Source: CAD feature listing. Evaluate the final solid. Frame: model axes, mm. A direction names the side the tool comes from. Give positions to 0.01 mm unless a question says otherwise; leave off trailing zeros. Order: outer loops, then holes, each group sorted by start corner. A loop starts at its lowest first (then second) coordinate and runs counter-clockwise, first axis right, second up.
Autodesk Inventor part; units mm, degrees
ref_plane "Plano de trabajo4" through (-2.7452, -1.596, 0) normal (0, 0, -1) x (-1, 0, 0)
ref_plane "Plano de trabajo5" through (0, -3.175, 0) normal (0, 1, 0) x (-1, 0, 0)
ref_plane "Barreno" through (0, 0, 0) normal (0, -1, 0) x (1, 0, 0)
sketch "Boceto1" plane through (0, 0, 0) normal (0, 0, 1) x (1, 0, 0)
  line L0 (2.7452, 1.596) -> (2.7548, -1.5794)
  line L1 (2.7548, -1.5794) -> (0.0096, -3.1754)
  line L2 (0.0096, -3.1754) -> (-2.7452, -1.596)
  line L3 (-2.7452, -1.596) -> (-2.7548, 1.5794)
  line L4 (-2.7548, 1.5794) -> (-0.0096, 3.1754)
  line L5 (-0.0096, 3.1754) -> (2.7452, 1.596)
  point P0 (0, 0)
  point P1 (0, 0)
  dimension "d0" = 5.5
  dimension "d20" = 6.3508
extrude "Extrusión1" add sketch "Boceto1" along normal blind 15
ref_plane "Plano de trabajo4" through (-2.7452, -1.596, 0) normal (0, 0, -1) x (-1, 0, 0)
sketch "Boceto2" plane through (-2.7452, -1.596, 0) normal (0, 0, -1) x (-1, 0, 0)
  line L0 (-2.7548, -1.5794) -> (1.0358, -1.5794)
  line L1 (1.0358, -1.5794) -> (-2.7548, -1.5794)
  line L2 (-5.6299, -1.5794) -> (-2.7548, -1.5794)
  point P0 (-2.7452, 1.596)
  dimension "d5" = 3.1754
ref_plane "Plano de trabajo5" through (0, -3.175, 0) normal (0, 1, 0) x (-1, 0, 0)
sketch "Boceto3" plane through (0, -3.175, 0) normal (0, 1, 0) x (-1, 0, 0)
  line L0 (-0.0096, 15) -> (-2.7548, 15)
  line L1 (2.6199, 14) -> (-2.7548, 14) construction
  line L2 (-0.0096, 0) -> (-0.0096, 15)
  line L3 (-0.0096, 14) -> (-0.0096, 18.5)
  circle A0 centre (-0.0096, 18.5) radius 4.25
  circle A1 centre (-0.0096, 18.5) radius 2.75
  point P0 (0, 0)
  dimension "d7" = 1
  dimension "d8" = 4.5
  dimension "d9" = 8.5
  dimension "d14" = 5.5
sketch "Boceto4" plane through (-2.7452, -1.596, 0) normal (0, 0, -1) x (-1, 0, 0)
  point P0 (-2.7452, 1.596)
  point P1 (-2.7356, 4.7714)
  point P2 (-2.7548, -1.579)
  dimension "d10" = 6.3504
extrude "Extrusión2" add sketch "Boceto3" along normal blind 6.35 contours L2 A0 L0 | L0 A0 L2 | A1
ref_plane "Barreno" through (0, 0, 0) normal (0, -1, 0) x (1, 0, 0)
sketch "Boceto6" plane through (0, 0, 0) normal (0, -1, 0) x (1, 0, 0)
  arc A0 (0.0103, 14.25) -> (0.0089, 14.25) centre (0.0096, 18.5) ccw
  circle A1 centre (0.0096, 18.5) radius 2.75
  point P0 (0, 0)
  dimension "d13" = 4.25
extrude "Extrusión3" cut sketch "Boceto6" along normal mid plane 10 contours A1
ref_plane "Plano de trabajo8" through (5, 0, 0) normal (1, 0, 0) x (0, 1, 0)
sketch "Boceto8" plane through (5, 0, 0) normal (1, 0, 0) x (0, 1, 0)
  line L0 (-3.175, 15.75) -> (-3.175, 21.25)
  line L1 (-3.1754, 14.25) -> (-1.5794, 15)
  line L2 (-1.5794, 15) -> (-1.5794, 22.75)
  line L3 (-1.5794, 22.75) -> (-3.175, 22.75)
  line L4 (3.175, 14.25) -> (1.596, 15)
  line L5 (1.596, 15) -> (1.596, 22.75)
  line L6 (1.596, 22.75) -> (3.175, 22.75)
  ellipse E0 centre (3.1866, 18.5) end of major axis (3.1866, 14.25) minor radius 2.4709 (1.7849, 15) -> (3.175, 14.25) ccw
  line L7 (-3.175, 22.75) -> (-6.1952, 22.75)
  line L8 (-6.1952, 22.75) -> (-6.1952, 14.0055)
  line L9 (-6.1952, 14.0055) -> (-3.1754, 14.25)
  line L10 (3.175, 14.25) -> (7.2865, 13.4418)
  line L11 (7.2865, 13.4418) -> (6.5328, 22.75)
  line L12 (6.5328, 22.75) -> (3.175, 22.75)
  point P0 (0, 0)
  point P1 (-1.5794, 15)
extrude "Extrusión4" cut sketch "Boceto8" against normal blind 10 contours L9 L8 L7 L3 L2 L1 | L4 L5 L6 L12 L11 L10
fillet "Empalme1" radius 2 1 edges at (-2.75, 0, 15)
fillet "Empalme2" radius 2 1 edges at (2.75, 0.0083, 15)
ref_plane "Plano de trabajo9" through (0, 0, 0) normal (0, 0, -1) x (-1, 0, 0)
sketch "Boceto9" plane through (0, 0, 0) normal (0, 0, -1) x (-1, 0, 0)
  circle A0 centre (0, 0) radius 2.75
  line L0 (2.7548, 1.5794) -> (2.7452, -1.596)
extrude "Extrusión5" add sketch "Boceto9" along normal blind 0.01
properties part number "Cabezal" material "Plástico ABS"
1) Section query A-A, the plane z = 18.5. Return the cut outline in (x, y).
Report:
outline: (-4.24, -1.58) - (-2.74, -1.58) - (-2.74, 1.6) - (-4.24, 1.6) - close; (2.76, -1.58) - (4.26, -1.58) - (4.26, 1.6) - (2.76, 1.6) - close
2) Section query D-D, the plane z = 4.5. Return the cut outline in (x, y), and give its area (3 significant figures).
Report:
outline: (-2.75, -1.6) - (0.01, -3.18) - (2.75, -1.58) - (2.75, 1.6) - (-0.01, 3.18) - (-2.75, 1.58) - close
area: 26.2 mm2
3) Pin query (flat end, axial travel): pin 1 (3.5 mm diameter, centred on x = 0.01, z = 18.5, fed in from +Y). Return the tip coordinate at first contact, or that it passes through.
Report:
pin 1: passes through
4) Reachability of faces 1 (the flat face through (-1.349, -2.397, 7.353)), 2 (the flat face through (1.349, 2.397, 7.358)), 3 (the flat face through (-1.401, 2.366, 7.358)), 4 (the flat face through (0.1, -1.579, 21.4)) from +Z, -Z, +X, -X, +Y, -Y: full face, straight path, thin tool, end or side. Return the list, or none.
Report:
face 1: -Z, -X, -Y
face 2: -Z, +X, +Y
face 3: -Z, -X, +Y
face 4: +Z, +X, -X, -Y
5) Material intervals for L1, parallel to Z at x = 0, y = -0.75; L2, parallel to X at y = -1, z = 13; L3, parallel to Z at x = 3.25, y = -1.5, sorted ascending.
Report:
L1: z = -0.01 to 15.75, 21.25 to 22.75
L2: x = -2.75 to 2.75
L3: z = 15.75 to 21.25
6) Section query C-C, the plane x = 0.5. Return the cut outline in (y, z) (3 decimals).
Report:
outline: (-3.115, 14.278) - (-2.89, 14.278) - (-2.89, 0) - (-2.704, 0) - (-2.704, -0.01) - (2.704, -0.01) - (2.704, 0) - (2.883, 0) - (2.883, 14.278) - (3.115, 14.278) - (1.596, 15) - (1.596, 15.794) - (-1.579, 15.794) - (-1.579, 15) - close; (-1.579, 21.206) - (1.596, 21.206) - (1.596, 22.722) - (-1.579, 22.722) - close
